Verification items for the finished model (mm, model axes). Face numbers are marked on the shaded views. A direction names the side the tool comes from. Coordinates: 2 decimals unless noted, no trailing zeros. Loops run counter-clockwise (first coordinate to the right, second up) from the corner with the lowest first, then second, coordinate; pieces in that order, holes last.
Q1. Sectioned sample at A-A (z = 0). Enter the section's corners in (x, y).
Q2. Sectioned sample at B-B (y = 22.5). Enter the section's corners in (x, z).
Q3. Material ranges on probe 1 along Z at (x, y) = (-22.5, 13); probe 2 along X at (y, z) = (7, 0); probe 3 along Y at (x, z) = (-9.5, 4.5), recorded low to high.
Q4. Go/stop test with flat-tipped pins: P1, Ø7.5, axis at y = 15, z = 0.5, coming from the -X side; P2, Ø4.5, axis at x = -9.5, y = 34.5, coming from the +Z side. Record where each tip stops, or that it passes through.
Q5. Access from +Z, -Z, +X, -X, +Y, -Y to the whole of each face (thin tool, end or side, straight path). Record for the marked faces 4, 5 and 6.
Q6. Sectioned sample at C-C (z = -10.5). Enter the section's corners in (x, y).
Q7. Mould release check, pull along Z, two halves, no side actions. Record for the marked faces 1, 2 and 3: +Z half, -Z half, draft (parallel to the pull), parting line (faces both ways), or undercut.
Q8. Sectioned sample at D-D (y = 11.5). Count the separate pieces of the cut face and the enclosed holes in it, then the cut area to 3 significant figures.
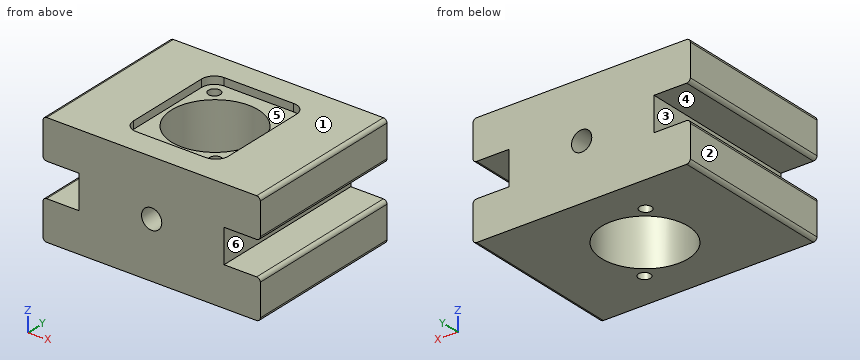
```python
from build123d import *

# Parameters (mm, degrees)
SKETCH1_R           = 2.8
BOSS_EXTRUDE1_DEPTH = 45
SKETCH2_R           = 12
SKETCH2_R_2         = 1.65
CUT_EXTRUDE1_DEPTH  = 56
CUT_EXTRUDE2_DEPTH  = 2.1


with BuildPart() as part:
    # Sketch1 → Boss-Extrude1 (new body)
    with BuildSketch(Plane(origin=(0, 0, 0), x_dir=(1, 0, 0), z_dir=(0, 1, 0))):
        with BuildLine():
            Line((20, -4.65), (20, 4.65))
            Line((20, 4.65), (29, 4.65))
            ThreePointArc((29, 4.65), (29.707106781, 4.942893219), (30, 5.65))
            Line((30, 5.65), (30, 14.5))
            ThreePointArc((30, 14.5), (29.707106781, 15.207106781), (29, 15.5))
            Line((29, 15.5), (20, 15.5))
            Line((20, 15.5), (-20, 15.5))
            Line((-20, 15.5), (-29, 15.5))
            ThreePointArc((-29, 15.5), (-29.707106781, 15.207106781), (-30, 14.5))
            Line((-30, 14.5), (-30, 5.65))
            ThreePointArc((-30, 5.65), (-29.707106781, 4.942893219), (-29, 4.65))
            Line((-29, 4.65), (-20, 4.65))
            Line((-20, 4.65), (-20, -4.65))
            Line((-20, -4.65), (-29, -4.65))
            ThreePointArc((-29, -4.65), (-29.707106781, -4.942893219), (-30, -5.65))
            Line((-30, -5.65), (-30, -14.5))
            ThreePointArc((-30, -14.5), (-29.707106781, -15.207106781), (-29, -15.5))
            Line((-29, -15.5), (-20, -15.5))
            Line((-20, -15.5), (20, -15.5))
            Line((20, -15.5), (29, -15.5))
            ThreePointArc((29, -15.5), (29.707106781, -15.207106781), (30, -14.5))
            Line((30, -14.5), (30, -5.65))
            ThreePointArc((30, -5.65), (29.707106781, -4.942893219), (29, -4.65))
            Line((29, -4.65), (20, -4.65))
        make_face()
        with Locations(Location((0, 0, 0), (0, 0, 90))):
            Circle(SKETCH1_R, mode=Mode.SUBTRACT)
    extrude(amount=BOSS_EXTRUDE1_DEPTH)

    # Sketch2 → Cut-Extrude1 (cut)
    with BuildSketch(Plane.XY.offset(15.5)):
        with Locations((0, 22.5)):
            Circle(SKETCH2_R)
        with Locations((-9.5, 34.5)):
            Circle(SKETCH2_R_2)
        with Locations((9.5, 10.5)):
            Circle(SKETCH2_R_2)
    extrude(amount=-CUT_EXTRUDE1_DEPTH, mode=Mode.SUBTRACT)

    # Sketch3 → Cut-Extrude2 (cut)
    with BuildSketch(Plane.XY.offset(15.5)):
        with BuildLine():
            Line((-9.6, 38.1), (9.6, 38.1))
            ThreePointArc((9.6, 38.1), (12.074873734, 37.074873734), (13.1, 34.6))
            Line((13.1, 34.6), (13.1, 10.4))
            ThreePointArc((13.1, 10.4), (12.074873734, 7.925126266), (9.6, 6.9))
            Line((9.6, 6.9), (-9.6, 6.9))
            ThreePointArc((-9.6, 6.9), (-12.074873734, 7.925126266), (-13.1, 10.4))
            Line((-13.1, 10.4), (-13.1, 34.6))
            ThreePointArc((-13.1, 34.6), (-12.074873734, 37.074873734), (-9.6, 38.1))
        make_face()
    extrude(amount=-CUT_EXTRUDE2_DEPTH, mode=Mode.SUBTRACT)


solid = part.part
```
Geometry check:
1. outline: (-20, 0) - (-2.8, 0) - (-2.8, 10.83) arc R12 cw to (-2.8, 34.17) - (-2.8, 45) - (-20, 45) - close; (2.8, 0) - (20, 0) - (20, 45) - (2.8, 45) - (2.8, 34.17) arc R12 cw to (2.8, 10.83) - close; hole circle Ø3.3 at (-9.5, 34.5); hole circle Ø3.3 at (9.5, 10.5)
2. outline: (-30, -14.5) arc R1 ccw to (-29, -15.5) - (-12, -15.5) - (-12, 13.4) - (-13.1, 13.4) - (-13.1, 15.5) - (-29, 15.5) arc R1 ccw to (-30, 14.5) - (-30, 5.65) arc R1 ccw to (-29, 4.65) - (-20, 4.65) - (-20, -4.65) - (-29, -4.65) arc R1 ccw to (-30, -5.65) - close; (12, -15.5) - (29, -15.5) arc R1 ccw to (30, -14.5) - (30, -5.65) arc R1 ccw to (29, -4.65) - (20, -4.65) - (20, 4.65) - (29, 4.65) arc R1 ccw to (30, 5.65) - (30, 14.5) arc R1 ccw to (29, 15.5) - (13.1, 15.5) - (13.1, 13.4) - (12, 13.4) - close
3. probe 1: z = -15.5 to -4.65, 4.65 to 15.5
3. probe 2: x = -20 to -2.8, 2.8 to 20
3. probe 3: y = 0 to 15.17, 29.83 to 32.85, 36.15 to 45
4. P1: stops at x = -20
4. P2: stops at z = 13.4
5. face 4: -X, +Y, -Y
5. face 5: +Z
5. face 6: +X, +Y, -Y
6. outline: (-30, 0) - (30, 0) - (30, 45) - (-30, 45) - close; hole circle Ø24 at (0, 22.5); hole circle Ø3.3 at (-9.5, 34.5); hole circle Ø3.3 at (9.5, 10.5)
7. face 1: +Z half
7. face 2: draft
7. face 3: undercut
8. separate pieces: 3
8. enclosed holes: 0
8. area: 1,260 mm2
